Check sheet for the modelled part. Datum: model origin and axes. Units: mm. A direction names the side the tool comes from. Coordinates: 2 decimals unless noted, no trailing zeros. Loops run counter-clockwise (first coordinate to the right, second up) from the corner with the lowest first, then second, coordinate; pieces in that order, holes last. Notation, with made-up numbers: M 24,-13 L 79,-13 A18 cw 79,7 Z; hole C 30.25,-15.75 d1. An arc over 180 degrees is marked long. Return JSON: item names as keys, results as strings.
from build123d import *

# Parameters (mm, degrees)
F2_W     = 19.995908
F2_H     = 19.98147
F3_DEPTH = 3
F4_DEPTH = 5
F5_R     = 1
F6_R     = 2
F7_R     = 2


with BuildPart() as f3:
    # F2 (on Top) → F3 (new body)
    with BuildSketch(Plane.XY):
        Rectangle(F2_W, F2_H)
    extrude(amount=F3_DEPTH)

    # F1 (on Top) → F4 (join)
    with BuildSketch(Plane.XY):
        Polygon((-8.5, 6.008047), (-8.5, -5.991953), (-7, -5.991953), (-4.5, -3.491953), (-4.5, 3.508047), (-7, 6.008047), align=None)
        Polygon((6, 8.508047), (-6, 8.508047), (-6, 7.008047), (-3.5, 4.508047), (3.5, 4.508047), (6, 7.008047), align=None)
        Polygon((7, -5.991953), (8.5, -5.991953), (8.5, 6.008047), (7, 6.008047), (4.5, 3.508047), (4.5, -3.491953), align=None)
        Polygon((-6, -6.991953), (-6, -8.491953), (6, -8.491953), (6, -6.991953), (3.5, -4.491953), (-3.5, -4.491953), align=None)
    extrude(amount=-F4_DEPTH)

    # F5
    f5_edges = [f3.edges().sort_by_distance(p)[0] for p in [
        (0, 8.508047, -5),
        (-6, 7.758047, -5),
        (-4.75, 5.758047, -5),
        (0, 4.508047, -5),
        (4.75, 5.758047, -5),
        (6, 7.758047, -5),
        (-5.75, 4.758047, -5),
        (-7.75, 6.008047, -5),
        (-8.5, 0.008047, -5),
        (-7.75, -5.991953, -5),
        (-5.75, -4.741953, -5),
        (-4.5, 0.008047, -5),
        (-6, -7.741953, -5),
        (0, -8.491953, -5),
        (6, -7.741953, -5),
        (4.75, -5.741953, -5),
        (0, -4.491953, -5),
        (-4.75, -5.741953, -5),
        (5.75, -4.741953, -5),
        (7.75, -5.991953, -5),
        (8.5, 0.008047, -5),
        (7.75, 6.008047, -5),
        (5.75, 4.758047, -5),
        (4.5, 0.008047, -5),
    ]]
    fillet(f5_edges, radius=F5_R)

    # F6
    f6_edges = [f3.edges().sort_by_distance(p)[0] for p in [
        (9.997954, 9.990735, 1.5),
        (9.997954, -9.990735, 1.5),
        (-9.997954, -9.990735, 1.5),
        (-9.997954, 9.990735, 1.5),
    ]]
    fillet(f6_edges, radius=F6_R)

    # F7
    f7_edges = [f3.edges().sort_by_distance(p)[0] for p in [
        (0, -9.990735, 3),
        (-9.412167, -9.404949, 3),
        (9.412167, -9.404949, 3),
        (-9.997954, 0, 3),
        (9.997954, 0, 3),
        (-9.412167, 9.404949, 3),
        (9.412167, 9.404949, 3),
        (0, 9.990735, 3),
    ]]
    fillet(f7_edges, radius=F7_R)


solid = f3.part
1) Section check D-D on z = 1.75. Record the cut outline in (x, y), then the cut area to 3 significant figures.
Answers:
{"outline": "M -9.85,-7.99 A1.85 ccw -8,-9.84 L 8,-9.84 A1.85 ccw 9.85,-7.99 L 9.85,7.99 A1.85 ccw 8,9.84 L -8,9.84 A1.85 ccw -9.85,7.99 Z", "area": "385 mm²"}
2) Set-up check for faces 1 (the face through (-7.76, 5.833, -4.565)), 2 (the face through (-6, -8, -2)), 3 (the face through (7.76, -5.82, -4.56)), 4 (the face through (-5.93, -4.52, -4.7)): record each of +Z, -Z, +X, -X, +Y, -Y from which the full face is reachable in a straight line by a thin tool's end or side.
Answers:
{"face 1": "-Z, -X, +Y", "face 2": "-Z, -X, -Y", "face 3": "-Z, +X, -Y", "face 4": "-Z"}
3) Go/stop test with flat-tipped pins: pin 1 Ø2 at (y, z) = (-1, -2) entering from +X; pin 2 Ø2 at (x, z) = (0, -2) entering from -Y; pin 3 Ø3 at (x, z) = (-2.5, -3) entering from +Y. Record where each tip stops, or that it passes through.
Answers:
{"pin 1": "x = 8.5", "pin 2": "y = -8.49", "pin 3": "y = 8.51"}
4) Draft check along X on faces 5 (the face through (6, 8, -2)), 6 (the face through (-4.5, 0, -2)), 7 (the face through (-9.998, -0.1, 0.5)). Enter one of: +X half, -X half, draft (parallel to the pull), parting line (faces both ways), or undercut.
Answers:
{"face 5": "+X half", "face 6": "undercut", "face 7": "-X half"}
5) Scan lines: line 1 along Y through (x, z) = (2.25, -0.5); line 2 along Y through (x, z) = (-4, -3.5); line 3 along X through (y, z) = (-5, -1). Record each from-to range of solid material in increasing order. Write a range as [from, to].
Answers:
{"line 1": "[-8.49, -4.49], [4.51, 8.51]", "line 2": "[-8.49, -4.99], [5.01, 8.51]", "line 3": "[-8.5, -6.01], [-4.01, 4.01], [6.01, 8.5]"}
6) Section check B-B on x = 1.5. Record the cut outline in (y, z).
Answers:
{"outline": "M -9.99,0 L -8.49,0 L -8.49,-4 A1 ccw -7.49,-5 L -5.49,-5 A1 ccw -4.49,-4 L -4.49,0 L 4.51,0 L 4.51,-4 A1 ccw 5.51,-5 L 7.51,-5 A1 ccw 8.51,-4 L 8.51,0 L 9.99,0 L 9.99,1 A2 ccw 7.99,3 L -7.99,3 A2 ccw -9.99,1 Z"}
7) Section check C-C on y = 1. Record the cut outline in (x, z).
Answers:
{"outline": "M -10,0 L -8.5,0 L -8.5,-4 A1 ccw -7.5,-5 L -5.5,-5 A1 ccw -4.5,-4 L -4.5,0 L 4.5,0 L 4.5,-4 A1 ccw 5.5,-5 L 7.5,-5 A1 ccw 8.5,-4 L 8.5,0 L 10,0 L 10,1 A2 ccw 8,3 L -8,3 A2 ccw -10,1 Z"}
8) Section check A-A on z = -1.75. Record the cut outline in (x, y), then the cut area to 3 significant figures.
Answers:
{"outline": "M -8.5,-5.99 L -7,-5.99 L -4.5,-3.49 L -4.5,3.51 L -7,6.01 L -8.5,6.01 Z; M -6,-8.49 L 6,-8.49 L 6,-6.99 L 3.5,-4.49 L -3.5,-4.49 L -6,-6.99 Z; M -6,7.01 L -3.5,4.51 L 3.5,4.51 L 6,7.01 L 6,8.51 L -6,8.51 Z; M 4.5,-3.49 L 7,-5.99 L 8.5,-5.99 L 8.5,6.01 L 7,6.01 L 4.5,3.51 Z", "area": "167 mm²"}
